The figure shows three views and two pictorial views of one solid part (mm, origin at its lowest corner). Answer the questions. Give positions to 0.01 mm unless a question says otherwise; leave off trailing zeros. One line per question, with ' | ' between items.
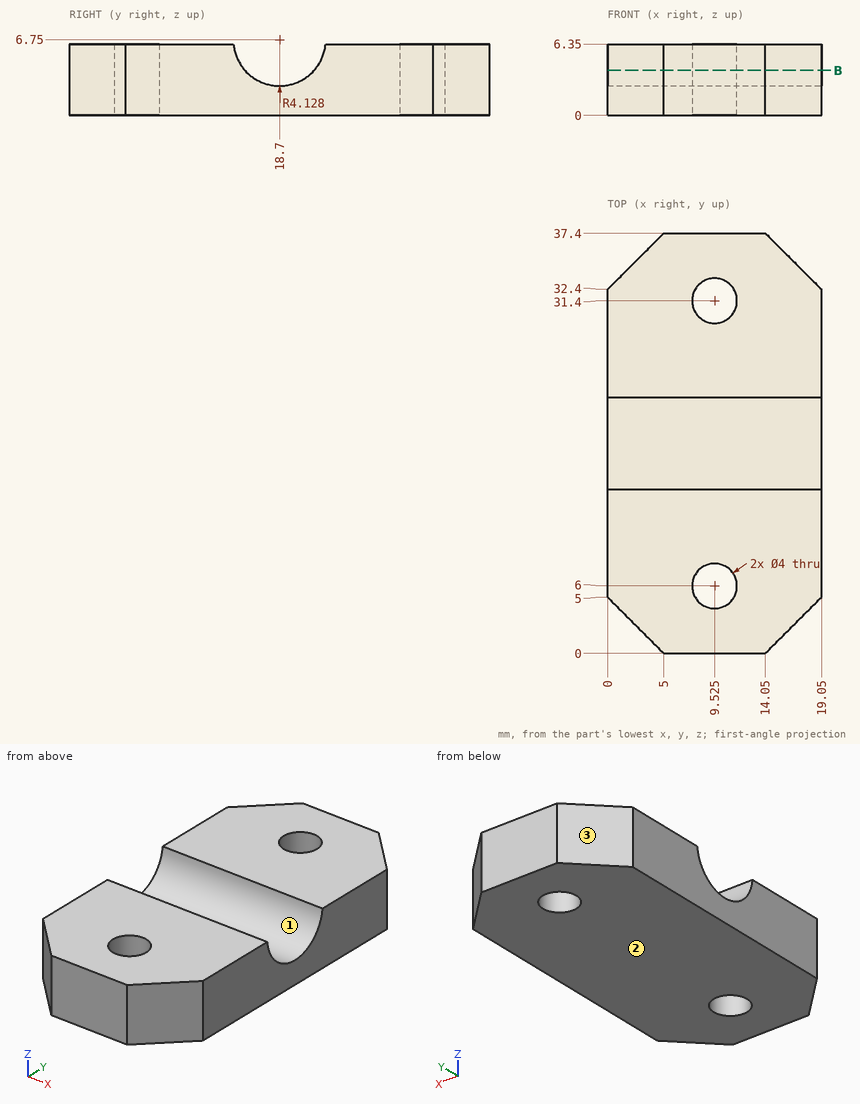
1. Consider L1, parallel to Y at x = 9.5, z = 1.5; L2, parallel to Y at x = 10, z = 4.25 (1 decimal); L3, parallel to Y at x = 9.25, z = 5. Determine where each line is inside the solid, lowest interval first.
Evaluation:
L1: 0 to 4, 8 to 29.4, 33.4 to 37.4 | L2: 0 to 4.1, 7.9 to 15.4, 22 to 29.5, 33.3 to 37.4 | L3: 0 to 4.02, 7.98 to 14.96, 22.44 to 29.42, 33.38 to 37.4
2. Determine the mould class of the marked faces 1, 2 and 3 for opening direction Y: +Y half, -Y half, draft (parallel to the pull), parting line (faces both ways), or undercut.
Evaluation:
face 1: undercut | face 2: draft | face 3: +Y half
3. Find section B-B on z = 4. State how many separate pieces and enclosed holes the cut face has, then the cut area to 3 significant figures.
Evaluation:
separate pieces: 2 | enclosed holes: 2 | area: 520 mm2
